```python
from build123d import *

# Parameters (mm, degrees)
SKETCH1_R           = 7.95
SKETCH1_R_2         = 1.5
SKETCH1_R_3         = 1.2
SKETCH1_W           = 8
SKETCH1_H           = 2.4
BOSS_EXTRUDE1_DEPTH = 5
CUT_EXTRUDE1_DEPTH  = 6


with BuildPart() as part:
    # Sketch1 → Boss-Extrude1 (new body)
    with BuildSketch(Plane(origin=(0, 0, 0), x_dir=(0, 0, -1), z_dir=(1, 0, 0))):
        Polygon((-50, 0), (0, 0), (0, 24), (-5, 24), (-5, 49), (0, 49), (0, 64), (-50, 64), (-50, 53), (-45, 53), (-45, 47), (-50, 47), (-50, 40), (-55, 40), (-55, 25), (-50, 25), align=None)
        with Locations((-20, 17)):
            Circle(SKETCH1_R, mode=Mode.SUBTRACT)
        with Locations((-45, 7.5)):
            Circle(SKETCH1_R_2, mode=Mode.SUBTRACT)
        with Locations((-32, 7.5)):
            Circle(SKETCH1_R_2, mode=Mode.SUBTRACT)
        with Locations((-2.5, 56.5)):
            Circle(SKETCH1_R_3, mode=Mode.SUBTRACT)
        with Locations((-2.5, 12)):
            Circle(SKETCH1_R_3, mode=Mode.SUBTRACT)
        with Locations((-38.5, 18.2)):
            Rectangle(SKETCH1_W, SKETCH1_H, mode=Mode.SUBTRACT)
    extrude(amount=BOSS_EXTRUDE1_DEPTH)

    # Sketch2 → Cut-Extrude1 (cut, through all)
    with BuildSketch(Plane(origin=(5, 0, 0), x_dir=(0, 0, -1), z_dir=(1, 0, 0))):
        Polygon((-50, 56.8), (-46, 56.8), (-46, 55.25), (-44.2, 55.25), (-44.2, 56.8), (-42.2, 56.8), (-42.2, 59.2), (-44.2, 59.2), (-44.2, 60.75), (-46, 60.75), (-46, 59.2), (-50, 59.2), align=None)
        Polygon((-44.2, 19.4), (-42.2, 19.4), (-42.2, 17), (-44.2, 17), (-44.2, 15.45), (-46, 15.45), (-46, 17), (-50, 17), (-50, 19.4), (-46, 19.4), (-46, 20.95), (-44.2, 20.95), align=None)
    extrude(amount=-CUT_EXTRUDE1_DEPTH, mode=Mode.SUBTRACT)


solid = part.part
```
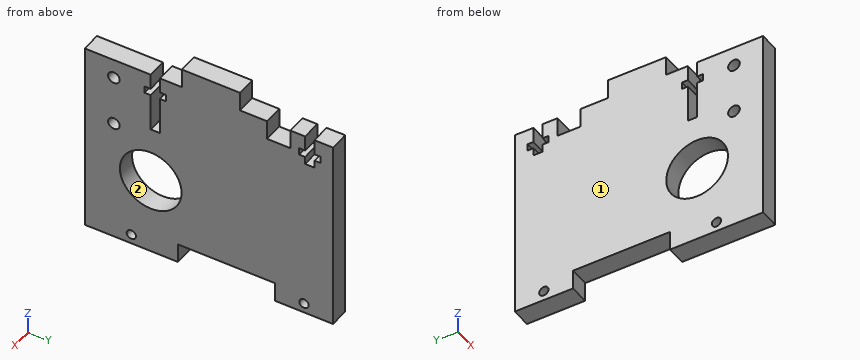
Check sheet for the modelled part. Datum: model origin and axes. Units: mm. Face numbers are marked on the shaded views. Round coordinates to 2 decimals unless told otherwise and drop trailing zeros. Order: outer loops, then holes, each group sorted by start corner. A loop starts at its lowest first (then second) coordinate and runs counter-clockwise, first axis right, second up. Notation, with made-up numbers: (2, -37) -> (51, -37) arc R10 ccw to (51, -25) -> close; hole circle Ø3 at (-32.5, -1). An arc over 180 degrees is marked (long way). One line per item, written item: value. Start each with the question number.
Q1. Cross-section at A-A (z = 32). Record the boundary of the cut face in (x, y), and give its area (3 significant figures).
Q2. Cross-section at B-B (y = 12). Record the boundary of the cut face in (x, z), and give its area (3 significant figures).
Q3. Cross-section at C-C (z = 41). Record the boundary of the cut face in (x, y).
Q4. Mould release check, pull along Z, two halves, no side actions. Record for the marked faces 1 and 2: pulls with the +Z half, pulls with the -Z half, needs draft (parallel to the pull), parting line crosses it, or undercut.
Q5. Thickness scan on line 1 (Y direction, x = 3.6, z = 2.5); line 2 (Y direction, x = 2.95, z = 20); line 3 (Z direction, x = 0.6, y = 7). Record the ranges inside material, lowest first.
Q6. Cross-section at D-D (x = 1.1). Give the number of separate pieces and of enclosed holes in the cut face, and give its area (3 significant figures).
Q7. Gauge pin test, flat ends, axial feed: pin 1 Ø2 at (x, z) = (3, 43) entering from -Y; pin 2 Ø2.5 at (x, z) = (2, 51.5) entering from +Y; pin 3 Ø1.5 at (x, y) = (2.5, 21) entering from +Z; pin 4 Ø0.7 at (x, y) = (3.5, 18.5) entering from +Z. Record the tip position at first contact, or that the pin passes through.
Completed:
1. outline: (0, 0) -> (5, 0) -> (5, 6) -> (0, 6) -> close; (0, 9) -> (5, 9) -> (5, 64) -> (0, 64) -> close
1. area: 305 mm²
2. outline: (0, 0) -> (5, 0) -> (5, 1.3) -> (0, 1.3) -> close; (0, 3.7) -> (5, 3.7) -> (5, 13.82) -> (0, 13.82) -> close; (0, 26.18) -> (5, 26.18) -> (5, 50) -> (0, 50) -> close
2. area: 176 mm²
3. outline: (0, 0) -> (5, 0) -> (5, 17) -> (0, 17) -> close; (0, 19.4) -> (5, 19.4) -> (5, 64) -> (0, 64) -> close
4. face 1: needs draft
4. face 2: undercut
5. line 1: y = 0 to 10.8, 13.2 to 24, 49 to 55.3, 57.7 to 64
5. line 2: y = 0 to 9.05, 24.95 to 64
5. line 3: z = 0 to 30.59, 33.41 to 43.59, 46.41 to 50
6. separate pieces: 1
6. enclosed holes: 5
6. area: 2,830 mm²
7. pin 1: stops at y = 0
7. pin 2: stops at y = 40
7. pin 3: stops at z = 50
7. pin 4: stops at z = 34.5
